Work out the finished part from the listing and answer in its coordinate system (mm). Face numbers are marked on the shaded views. Coordinates: 2 decimals unless noted, no trailing zeros. Order: outer loops, then holes, each group sorted by start corner. A loop starts at its lowest first (then second) coordinate and runs counter-clockwise, first axis right, second up. Notation, with made-up numbers: (40, -22) -> (64, -22) arc R26 ccw to (64, 4) -> close; hole circle Ø10 at (40, 34.25). An arc over 180 degrees is marked (long way). Answer as CSV lines item,"result". Start each with the question number.
Item 1: For a pull along Y with two mould halves and no side action, classify the marked faces 1, 2 and 3 as pulls with the +Y half, pulls with the -Y half, needs draft (parallel to the pull), parting line crosses it, or undercut.
Item 2: Section A-A (z = 0) is taken. Write down the section's boundary in (x, y), then the cut area to 3 significant figures.
Item 3: Section B-B (x = -2) is taken. Write down the section's boundary in (y, z), then the cut area to 3 significant figures.
Item 4: Straight lines are drawn through the part: L1, parallel to Z at x = -0.8, y = 3.75; L2, parallel to Y at x = -0.7, z = 0.5; L3, parallel to Y at x = -2.8, z = -3.75. For each, find the intervals that lie inside material, in ascending order.
Item 5: Each of these flat-tipped pins is pushed along its axis until it touches: pin 1 Ø1 at (x, y) = (-0.5, 5) entering from -Z; pin 2 Ø1.5 at (x, z) = (-1, -1) entering from +Y; pin 3 Ø1 at (x, y) = (-1.5, 5.5) entering from +Z. Where does it stop, or does it pass through?
```python
from build123d import *

# Parameters (mm, degrees)
SKETCH_2_W          = 3
SKETCH_2_H          = 7
SKETCH_3_R          = 1.25
CUT_EXTRUDE_1_DEPTH = 11.344080433
CHAMFER_1_SIZE      = 0.4


with BuildPart() as part:
    # Эскиз2 → Повернуть1 (revolve)
    with BuildSketch(Plane.XY, mode=Mode.PRIVATE) as revolve_1_sk:
        with Locations((-1.5, 3.5)):
            Rectangle(SKETCH_2_W, SKETCH_2_H)
    revolve(revolve_1_sk.sketch.rotate(Axis((-3, 0, 0), (1, 0, 0)), 180), axis=Axis((-3, 0, 0), (1, 0, 0)))

    # Эскиз3 → Вырез-Вытянуть1 (cut, through all)
    with BuildSketch(Plane.ZY.offset(3)):
        with Locations((0, 4)):
            Circle(SKETCH_3_R)
    extrude(amount=-CUT_EXTRUDE_1_DEPTH, mode=Mode.SUBTRACT)

    # Фаска1
    chamfer_1_edges = [part.edges().sort_by_distance(p)[0] for p in [
        (-3, 7, 0),
        (0, 7, 0),
    ]]
    chamfer(chamfer_1_edges, length=CHAMFER_1_SIZE)


solid = part.part
```
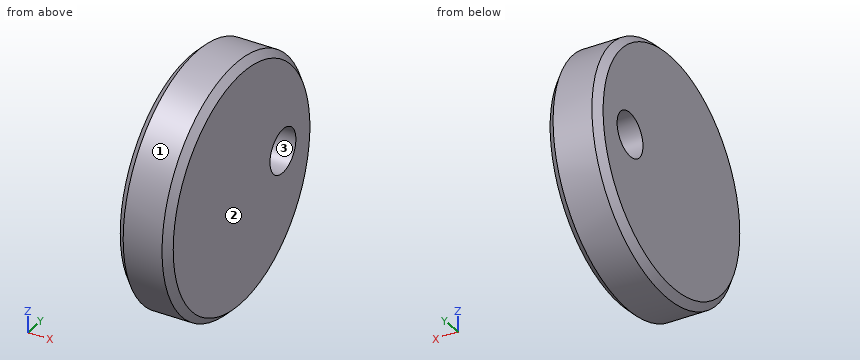
Checked values:
1,face 1,"parting line crosses it"
1,face 2,"needs draft"
1,face 3,"undercut"
2,outline,"(-3, -6.6) -> (-2.6, -7) -> (-0.4, -7) -> (0, -6.6) -> (0, 2.75) -> (-3, 2.75) -> close; (-3, 5.25) -> (0, 5.25) -> (0, 6.6) -> (-0.4, 7) -> (-2.6, 7) -> (-3, 6.6) -> close"
2,area,"34.2 mm^2"
3,outline,"circle Ø14 at (0, 0); hole circle Ø2.5 at (4, 0)"
3,area,"149 mm^2"
4,L1,"z = -5.91 to -1.22, 1.22 to 5.91"
4,L2,"y = -6.98 to 2.85, 5.15 to 6.98"
4,L3,"y = -5.67 to 5.67"
5,pin 1,"stops at z = -5.36"
5,pin 2,"stops at y = 7"
5,pin 3,"stops at z = 4.9"
